from build123d import *

# Parameters (mm, degrees)
SKETCH2_R                     = 19.0875
BOSS_EXTRUDE1_DEPTH           = 100
BOSS_EXTRUDE2_REACH           = 96.162
BOSS_EXTRUDE2_END_RADIUS      = 19.0875
SKETCH3_R                     = 19.0875
SHELL1_OUTLINE_R              = 17.5
SHELL1_DEPTH                  = 100
SHELL1_START                  = -37.059047745
SHELL1_2_OUTLINE_R            = 17.5
SHELL1_2_DEPTH                = 50.0000001
SKETCH6_W                     = 2.75
SKETCH6_H                     = 19.0875
M5_CLEARANCE_HOLE1_AT_2_COUNT = 2
M5_CLEARANCE_HOLE1_AT_2_PITCH = 44.503273363
MIRROR1_COPY_1_SKETCH_W       = 2.75
MIRROR1_COPY_1_SKETCH_H       = 19.0875
CUT_EXTRUDE1_START            = -30
SKETCH7_R                     = 19.0875
SKETCH7_R_2                   = 17.5
CUT_EXTRUDE1_DEPTH            = 30


with BuildPart() as part:
    # Sketch2 → Boss-Extrude1 (new body)
    with BuildSketch(Plane(origin=(0, 0, 0), x_dir=(0, 0, -1), z_dir=(1, 0, 0))):
        Circle(SKETCH2_R)
    extrude(amount=BOSS_EXTRUDE1_DEPTH)

    # Boss-Extrude2: up to this cylinder (the profile starts outside it)
    boss_extrude2_end = Plane(origin=(37.059048, 0, 0), z_dir=(-1, 0, 0)) * Cylinder(BOSS_EXTRUDE2_END_RADIUS, 231.499, mode=Mode.PRIVATE)
    # Sketch3 → Boss-Extrude2 (add, up to the surface)
    with BuildSketch(Plane(origin=(37.059047745, 0, 48.296291314), x_dir=(0.9659258262890673, 0, 0.2588190451025246), z_dir=(-0.2588190451025246, 0, 0.9659258262890673)), mode=Mode.PRIVATE) as boss_extrude2_sk1:
        Circle(SKETCH3_R)
    boss_extrude2_tool1 = extrude(boss_extrude2_sk1.sketch, amount=-BOSS_EXTRUDE2_REACH, mode=Mode.PRIVATE) - boss_extrude2_end
    add(boss_extrude2_tool1.solids().sort_by_distance((37.059048, 0, 48.296291))[0])

    # Shell1: read off the stored shape, not the designer's step
    # Shell1 outline → Shell1 (cut)
    with BuildSketch(Plane.YZ):
        Circle(SHELL1_OUTLINE_R)
    extrude(amount=SHELL1_DEPTH, mode=Mode.SUBTRACT)

    # Shell1 2 outline → Shell1 2 (cut)
    with BuildSketch(Plane(origin=(0, 0, 0), x_dir=(0.9659258262890672, 0, 0.2588190451025251), z_dir=(0.25881904510252507, 0, -0.9659258262890672)).offset(SHELL1_START)):
        with Locations((48.296291314, 0)):
            Circle(SHELL1_2_OUTLINE_R)
    extrude(amount=SHELL1_2_DEPTH, mode=Mode.SUBTRACT)

    # Sketch6 → M5 Clearance Hole1 (revolve, cut)
    with BuildSketch(Plane(origin=(15, 0, 0), x_dir=(0, 0, -1), z_dir=(1, 0, 0))):
        with Locations((1.375, 9.54375)):
            Rectangle(SKETCH6_W, SKETCH6_H)
    m5_clearance_hole1 = revolve(axis=Axis((15, -6.35, 0), (0, 1, 0)), mode=Mode.SUBTRACT)

    # M5 Clearance Hole1 at 2: M5 Clearance Hole1 ×2
    with Locations(*[Vector(0.5654612432844534, 0, 0.8247748676719001) * (i * M5_CLEARANCE_HOLE1_AT_2_PITCH) for i in range(1, M5_CLEARANCE_HOLE1_AT_2_COUNT)]):
        add(m5_clearance_hole1, mode=Mode.SUBTRACT)

    # Mirror1: M5 Clearance Hole1 across plane
    add(m5_clearance_hole1.mirror(Plane.ZX), mode=Mode.SUBTRACT)

    # Mirror1 copy 1 sketch → Mirror1 copy 1 (revolve, cut)
    with BuildSketch(Plane(origin=(40.164876286, 0, 36.705181399), x_dir=(0, 0, -1), z_dir=(1, 0, 0))):
        with Locations((1.375, -9.54375)):
            Rectangle(MIRROR1_COPY_1_SKETCH_W, MIRROR1_COPY_1_SKETCH_H)
    revolve(axis=Axis((40.164876286, 6.35, 36.705181399), (0, 1, 0)), mode=Mode.SUBTRACT)

    # Sketch7 → Cut-Extrude1 (cut)
    with BuildSketch(Plane(origin=(100, 0, 0), x_dir=(0, 0, -1), z_dir=(1, 0, 0)).offset(CUT_EXTRUDE1_START)):
        Circle(SKETCH7_R)
        Circle(SKETCH7_R_2, mode=Mode.SUBTRACT)
    extrude(amount=CUT_EXTRUDE1_DEPTH, mode=Mode.SUBTRACT)


solid = part.part
CAD build for the part. Positions are in the model's coordinates, mm. Round coordinates to 2 decimals unless told otherwise and drop trailing zeros. Order: outer loops, then holes, each group sorted by start corner. A loop starts at its lowest first (then second) coordinate and runs counter-clockwise, first axis right, second up. Notation, with made-up numbers: (56.25, 87) -> (60.25, 87) arc R23 cw to (60.25, 108) -> close; hole circle Ø4 at (37.25, 30.25). An arc over 180 degrees is marked (long way). Write each question's results on one line, items separated by ' | '.
1. Cut at D-D (y = 9). Give the cut face in (x, z), plus the area to 3 significant figures.
Findings below:
outline: (0, -16.83) -> (70, -16.83) -> (70, -15.01) -> (0, -15.01) -> close; (0, 15.01) -> (30.44, 15.01) -> (22.56, 44.41) -> (20.8, 43.94) -> (28.06, 16.83) -> (0, 16.83) -> close; (51.56, 52.18) -> (61.52, 15.01) -> (70, 15.01) -> (70, 16.83) -> (62.92, 16.83) -> (53.32, 52.65) -> close | area: 318 mm²
2. Wall check: line 1 along Y through (x, z) = (18, 0); line 2 along Y through (x, z) = (45, 44.5); line 3 along X through (y, z) = (-14, 20.5). Give the ranges that are in metal, low to high. Write a range as [from, to].
Findings below:
line 1: y = [-19.09, -17.5], [17.5, 19.09] | line 2: y = [-17.88, -16.17], [16.17, 17.88] | line 3: x = [31.08, 33.64], [55.38, 57.94]
3. Flat gauge pins, fed straight in: P1, Ø3.5, axis at x = 40.16, z = 36.71, coming from the +Y side; P2, Ø6, axis at x = 30, z = -5, coming from the +Y side; P3, Ø5, axis at x = 48, z = 19, coming from the +Y side; P4, Ø2, axis at y = 10, z = 32, coming from the -X side. Where does each tip first touch, or does it go through?
Findings below:
P1: passes through | P2: stops at y = 18.98 | P3: stops at y = 19.08 | P4: stops at x = 23.94
4. Pull direction X, two halves, no side cores. Call faces 1 (the face through (12.273, 18.198, 0.358)), 2 (the face through (70, -6, -17)), 3 (the face through (0, -6, -17)): pulls with the +X half, pulls with the -X half, needs draft (parallel to the pull), parting line crosses it, or undercut.
Findings below:
face 1: undercut | face 2: pulls with the +X half | face 3: pulls with the -X half
5. Cut at C-C (z = -9). Give the cut face in (x, y), plus the area to 3 significant figures.
Findings below:
outline: (0, -16.83) -> (70, -16.83) -> (70, -15.01) -> (0, -15.01) -> close; (0, 15.01) -> (70, 15.01) -> (70, 16.83) -> (0, 16.83) -> close | area: 255 mm²
6. Cut at B-B (y = 0). Give the cut face in (x, z).
Findings below:
outline: (0, -19.09) -> (70, -19.09) -> (70, -17.5) -> (0, -17.5) -> close; (0, 17.5) -> (27.19, 17.5) -> (20.16, 43.77) -> (18.62, 43.36) -> (25.12, 19.09) -> (0, 19.09) -> close; (53.96, 52.83) -> (63.43, 17.5) -> (70, 17.5) -> (70, 19.09) -> (64.65, 19.09) -> (55.5, 53.24) -> close
